Autodesk Inventor part; units mm, degrees
ref_plane "YZ Plane" through (0, 0, 0) normal (1, 0, 0) x (0, 1, 0)
ref_plane "XZ Plane" through (0, 0, 0) normal (0, 1, 0) x (-1, 0, 0)
ref_plane "XY Plane" through (0, 0, 0) normal (0, 0, 1) x (1, 0, 0)
sketch "Esquisse1" plane through (0, 0, 0) normal (0, 1, 0) x (-1, 0, 0)
  line L0 (0, 0) -> (50, 0)
  line L1 (50, 0) -> (50, -40)
  line L2 (50, -40) -> (0, -40)
  line L3 (0, -40) -> (0, 0)
  line L4 (50, -20) -> (0, -20) construction
  line L5 (50, -10) -> (0, -10) construction
  line L6 (50, -30) -> (0, -30) construction
  circle A0 centre (45, -5) radius 2.5
  line L7 (25, 0) -> (25, -40) construction
  circle A1 centre (5, -5) radius 2.5
  circle A2 centre (45, -35) radius 2.5
  circle A3 centre (5, -35) radius 2.5
  dimension "d0" = 50
  dimension "d2" = 10
  dimension "d3" = 10
  dimension "d4" = 5
  dimension "d12" = 5
  dimension "d13" = 20
  dimension "d14" = 20
extrude "Extrusion1" add sketch "Esquisse1" along normal blind 6
equation "\"d3\" = d2"
properties part number "hold_motor_bottom" material "Bois (cerisier)"
Can you work these out from the model? Positions are in its coordinate system, mm. Round coordinates to 2 decimals unless told otherwise and drop trailing zeros. Loops run counter-clockwise (first coordinate to the right, second up) from the corner with the lowest first, then second, coordinate; pieces in that order, holes last. Notation, with made-up numbers: M 25,63.5 L 81,63.5 A17 ccw 81,87.5 Z; hole C 41.5,-8.75 d4. An arc over 180 degrees is marked long. Answer as a JSON object with one key per item and string values. Group by question number.
Q1. Please list where these lines run through material, in increasing order: L1, parallel to Z at x = -45, y = 2.1; L2, parallel to Z at x = -44, y = 0.25.
Q2. We'd pull the mould along Z, two halves only. Please class faces 1 (the flat face through (-25, 3, -40)), 2 (the cylindrical face through (-47.31, 2.96, -4.04)), 3 (the flat face through (-50, 3, -20)): +Z half, -Z half, draft (parallel to the pull), parting line (faces both ways), or undercut.
Q3. Imagine slicing it at C-C, the plane y = 2.35. Please give me the cut outline in (x, z), then the cut area to 3 significant figures.
Q4. Imagine slicing it at B-B, the plane z = -5. Please give me the cut outline in (x, y).
Q5. Imagine slicing it at A-A, the plane x = -45. Please give me the cut outline in (y, z), then the cut area to 3 significant figures.
Findings:
{
 "1": {"L1": "z = -40 to -37.5, -32.5 to -7.5, -2.5 to 0", "L2": "z = -40 to -37.29, -32.71 to -7.29, -2.71 to 0"},
 "2": {"face 1": "-Z half", "face 2": "undercut", "face 3": "draft"},
 "3": {"outline": "M -50,-40 L 0,-40 L 0,0 L -50,0 Z; hole C -45,-35 d5; hole C -45,-5 d5; hole C -5,-35 d5; hole C -5,-5 d5", "area": "1,920 mm2"},
 "4": {"outline": "M -50,0 L -47.5,0 L -47.5,6 L -50,6 Z; M -42.5,0 L -7.5,0 L -7.5,6 L -42.5,6 Z; M -2.5,0 L 0,0 L 0,6 L -2.5,6 Z"},
 "5": {"outline": "M 0,-40 L 6,-40 L 6,-37.5 L 0,-37.5 Z; M 0,-32.5 L 6,-32.5 L 6,-7.5 L 0,-7.5 Z; M 0,-2.5 L 6,-2.5 L 6,0 L 0,0 Z", "area": "180 mm2"}
}
